Here's how the part is built. I have some questions about the finished solid (model axes, mm). Coordinates: 2 decimals unless noted, no trailing zeros. Order: outer loops, then holes, each group sorted by start corner. A loop starts at its lowest first (then second) coordinate and runs counter-clockwise, first axis right, second up. Notation, with made-up numbers: (47.5, -3.5) - (105.5, -3.5) arc R31 cw to (105.5, 35.5) - close; hole circle Ø4 at (64, 41). An arc over 180 degrees is marked (long way). Use CSV: the item, a comma, the result in double quotes. Start each with the question number.
from build123d import *

# Parameters (mm, degrees)
BOSS_EXTRUDE1_DEPTH = 6.35
SKETCH2_R           = 3.3782
CUT_EXTRUDE1_DEPTH  = 6.35


with BuildPart() as part:
    # Sketch1 → Boss-Extrude1 (new body)
    with BuildSketch(Plane.XY):
        with BuildLine():
            Line((-203.2, 228.6), (152.4, 228.6))
            ThreePointArc((152.4, 228.6), (188.321024484, 213.721024484), (203.2, 177.8))
            Line((203.2, 177.8), (203.2, -177.8))
            ThreePointArc((203.2, -177.8), (188.321024484, -213.721024484), (152.4, -228.6))
            Line((152.4, -228.6), (-50.8, -228.6))
            ThreePointArc((-50.8, -228.6), (-158.563073453, -183.963073453), (-203.2, -76.2))
            Line((-203.2, -76.2), (-203.2, 228.6))
        make_face()
    extrude(amount=BOSS_EXTRUDE1_DEPTH)

    # Sketch2 → Cut-Extrude1 (cut)
    with BuildSketch(Plane(origin=(0, 0, 0), x_dir=(-1, 0, 0), z_dir=(0, 0, -1))):
        with Locations((-81.049562296, 161.155935463)):
            Circle(SKETCH2_R)
        with Locations((-152.169562296, 180.205935019)):
            Circle(SKETCH2_R)
        with Locations((63.730437704, 154.805935463)):
            Circle(SKETCH2_R)
        with Locations((-12.469562296, 156.075935463)):
            Circle(SKETCH2_R)
    extrude(amount=-CUT_EXTRUDE1_DEPTH, mode=Mode.SUBTRACT)


solid = part.part
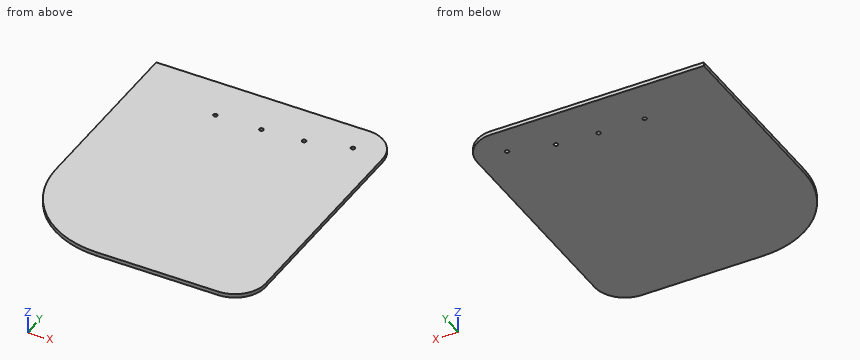
Item 1: Suppose I cut it at C-C on y = -135.5. Write out the boundary of the cut face in (x, z).
Item 2: For pin 1 Ø1.5 at (x, z) = (-150, 1.5) entering from -Y, with a flat end and sliding along its axis, tell me the tip position at first contact or that it passes through.
Item 3: Please list where these lines run through material, in increasing order: line 1 along Y through (x, z) = (152, 4.25); line 2 along X through (y, z) = (181, 1); line 3 along Y through (x, z) = (80.5, 1.5). Write a range as from..to.
Item 4: Suppose I cut it at A-A on x = -176.5. Write out the boundary of the cut face in (y, z), then the cut area to 3 significant figures.
Item 5: Suppose I cut it at B-B on z = 2.5. Write out the boundary of the cut face in (x, y).
Here are the results:
1,outline,"(-191.19, 0) - (203.2, 0) - (203.2, 6.35) - (-191.19, 6.35) - close"
2,pin 1,"y = -192.53"
3,line 1,"-228.6..176.83, 183.58..228.6"
3,line 2,"-203.2..148.89, 155.45..203.1"
3,line 3,"-228.6..157.82, 164.49..228.6"
4,outline,"(-162.37, 0) - (228.6, 0) - (228.6, 6.35) - (-162.37, 6.35) - close"
4,area,"2,480 mm^2"
5,outline,"(-203.2, -76.2) arc R152.4 ccw to (-50.8, -228.6) - (152.4, -228.6) arc R50.8 ccw to (203.2, -177.8) - (203.2, 177.8) arc R50.8 ccw to (152.4, 228.6) - (-203.2, 228.6) - close; hole circle Ø6.76 at (-63.73, 154.81); hole circle Ø6.76 at (12.47, 156.08); hole circle Ø6.76 at (81.05, 161.16); hole circle Ø6.76 at (152.17, 180.21)"
